Read the model definition and answer for the solid it produces. Units are mm, in the model's axes. Coordinates: 2 decimals unless noted, no trailing zeros. Write each loop counter-clockwise with the first axis right and the second up, starting at its lowest first coordinate (ties: lowest second). Pieces come first, ordered by that corner, then holes. Notation, with made-up numbers: M 20.25,78.5 L 46.25,78.5 A22 ccw 46.25,88.5 Z; hole C -3.75,51 d8. An arc over 180 degrees is marked long. Write item = value, one per line.
Autodesk Fusion 360 part; units mm, degrees
sketch "Esquisse1" plane through (0, 0, 0) normal (0, 0, 1) x (1, 0, 0)
  line L0 (0, 0) -> (250, 0)
  line L1 (250, 0) -> (250, 200)
  line L2 (250, 200) -> (0, 200)
  line L3 (0, 200) -> (0, 0)
  dimension "d18" = 200
  dimension "d19" = 250
extrude "Extrusion1" add sketch "Esquisse1" along normal blind 4
chamfer "Chanfrein1" distance 4 angle 45 1 faces at (83.3333, 133.3333, 0)
sketch "Esquisse2" plane through (0, 0, 4) normal (0, 0, 1) x (-1, 0, 0)
  circle A0 centre (-20, -180) radius 1.5
  circle A1 centre (-230, -180) radius 1.5
  circle A2 centre (-230, -20) radius 1.5
  circle A3 centre (-20, -20) radius 1.5
  line L0 (0, 0) -> (-20, -20)
  line L1 (-250, 0) -> (-230, -20)
  line L2 (-250, 0) -> (-297.1716, 0) construction
  line L3 (0, -200) -> (-20, -180)
  line L4 (-250, -200) -> (-230, -180)
  line L5 (-250, -200) -> (-297.1716, -200) construction
  line L6 (0, -200) -> (0, 0)
  line L7 (0, 0) -> (-250, 0)
  line L8 (-250, 0) -> (-250, -200)
  line L9 (-250, -200) -> (0, -200)
  dimension "d10" = 3
  dimension "d11" = 3
  dimension "d12" = 3
  dimension "d13" = 3
  dimension "d20" = 28.2843
  dimension "d22" = 45
  dimension "d23" = 28.2843
  dimension "d24" = 28.2843
  dimension "d25" = 28.2843
  dimension "d26" = 45
extrude "Extrusion2" cut sketch "Esquisse2" against normal blind 14 contours A0 | A3 | A2 | A1
thread "Filetage1" thread offset 0 thread length 10
thread "Filetage2" thread offset 0 thread length 10
thread "Filetage3" thread offset 0 thread length 10
thread "Filetage4" thread offset 0 thread length 10
equation "d20 = ( sqrt(800) ) * 1 mm"
equation "d23 = ( sqrt(800) ) * 1 mm"
equation "d24 = ( sqrt(800) ) * 1 mm"
equation "d25 = ( sqrt(800) ) * 1 mm"
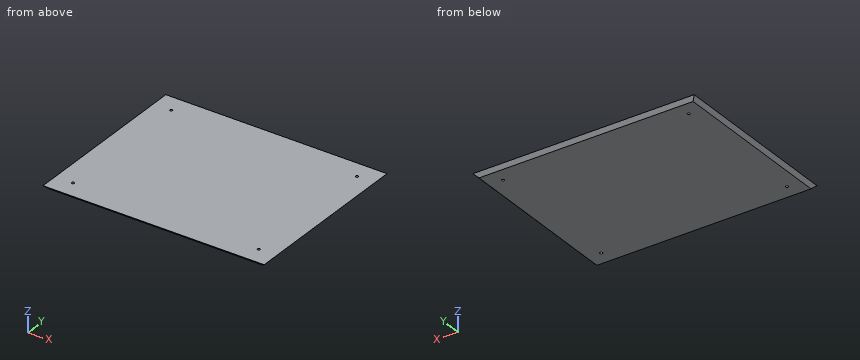
Item 1: Consider line 1 along X through (y, z) = (180, 0.85); line 2 along Y through (x, z) = (230, 3.15); line 3 along Y through (x, z) = (20, 1.7). Determine where each line is inside the solid, lowest interval first. Write a range as from..to.
Worked answers:
line_1 = 3.15..18.5, 21.5..228.5, 231.5..246.85
line_2 = 0.85..18.5, 21.5..178.5, 181.5..199.15
line_3 = 2.3..18.5, 21.5..178.5, 181.5..197.7
Item 2: Flat-ended cylindrical pins translate along their axes: pin 1 (5 mm diameter, centred on x = 224.5, y = 171, fed in from -Z); pin 2 (1 mm diameter, centred on y = 36, z = 2.5, fed in from -X); pin 3 (1.5 mm diameter, centred on y = 143, z = 1.5, fed in from -X). Find the tip coordinate at first contact, or state that the pin passes through.
Worked answers:
pin_1 = 0
pin_2 = 1
pin_3 = 1.75
Item 3: Find section A-A (z = 1). Determine the outline of the cut face in (x, y).
Worked answers:
outline = M 3,3 L 247,3 L 247,197 L 3,197 Z; hole C 20,20 d3; hole C 20,180 d3; hole C 230,20 d3; hole C 230,180 d3
